```python
from build123d import *

# Parameters (mm, degrees)
F1_DEPTH = 70
F3_DEPTH = 70.001
F5_DEPTH = 5
F7_DEPTH = 5
F6_R     = 2.5
F8_DEPTH = 6


with BuildPart() as f1:
    # F0 (on Front) → F1 (new body)
    with BuildSketch(Plane.XZ):
        Polygon((64.8236190979, 0), (70, 0), (63.1167820899, 25.6885189599), (39.1096145047, 115.2844881338), (34.2799853733, 113.9903929083), (36.2175250532, 106.7593963813), (0, 0), (5.2798833988, 0), (38.5474912469, 98.0638441664), align=None)
    extrude(amount=F1_DEPTH)

    # F2 (on Right) → F3 (cut, through all)
    with BuildSketch(Plane.YZ):
        Polygon((-31.1044628837, 176.4021748616), (0, 0), (48.4349839389, -5.1851687022), (65.811291337, 203.3304870129), align=None)
        Polygon((-111.5468591452, -12.9745472223), (-70, 0), (-38.8955371163, 176.4021748616), (-111.5468591452, 176.4021748616), align=None)
    extrude(amount=F3_DEPTH, mode=Mode.SUBTRACT)

    # F4 (on face) → F5 (cut)
    with BuildSketch(Plane(origin=(0, 0, 0), x_dir=(0, -1, 0), z_dir=(-0.9469906099, 0, 0.3212612407))):
        Polygon((58.1917434691, 10.0000029223), (42.7067823189, 102.7354300022), (27.2932176811, 102.7354300022), (11.8082565309, 10.0000029223), align=None)
    extrude(amount=-F5_DEPTH, mode=Mode.SUBTRACT)

    # F6 (on face) → F7 (cut)
    with BuildSketch(Plane(origin=(65.3108891325, 0, 17.5), x_dir=(0, 1, 0), z_dir=(0.9659258263, 0, 0.2588190451))):
        Polygon((-10.1440055617, -18.1173331572), (-11.8471934071, -8.1173331572), (-14.0249093092, 4.6687838175), (-55.9750906908, 4.6687838175), (-58.1528065929, -8.1173331572), (-59.8559944383, -18.1173331572), align=None)
        Polygon((-26.5845061685, 78.4104846719), (-43.4154938315, 78.4104846719), (-54.3229984458, 14.3687840231), (-15.6770015542, 14.3687840231), align=None)
    extrude(amount=-F7_DEPTH, mode=Mode.SUBTRACT)

    # F6 (on face) → F8 (join)
    with BuildSketch(Plane(origin=(65.3108891325, 0, 17.5), x_dir=(0, 1, 0), z_dir=(0.9659258263, 0, 0.2588190451))):
        with Locations((-60.195499549, 9.6687838175)):
            Circle(F6_R)
        with Locations((-9.804500451, 9.6687838175)):
            Circle(F6_R)
    extrude(amount=F8_DEPTH)


solid = f1.part
```
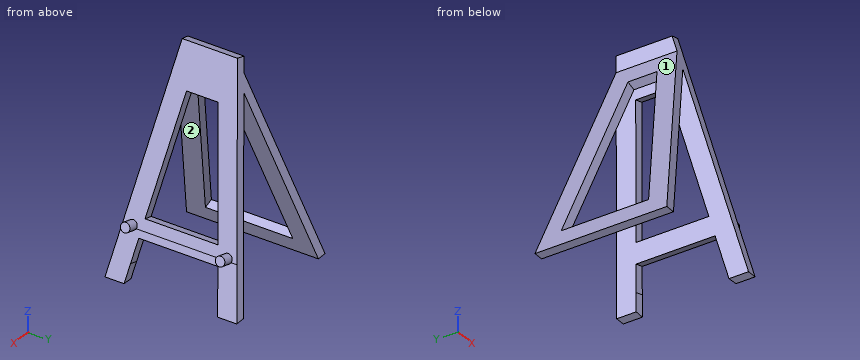
Build history of the part. All positions in model axes, mm. Face numbers are marked on the shaded views. Coordinates: 2 decimals unless noted, no trailing zeros. Order: outer loops, then holes, each group sorted by start corner. A loop starts at its lowest first (then second) coordinate and runs counter-clockwise, first axis right, second up. Notation, with made-up numbers: (67, 40.25) -> (88, 40.25) arc R19 cw to (88, 55.25) -> close; hole circle Ø6 at (1.5, 8.5). An arc over 180 degrees is marked (long way). Answer in a Markdown table with one row per item. Add a question column.
Q1. Band-saw the part on D-D, the plane x = 50.5. List the corners of the cut face in (y, z) (3 decimals), then the cut area to 3 significant figures.
Q2. Wall check: line 1 along X through (y, z) = (-46.5, 93); line 2 along X through (y, z) = (-19, 94); line 3 along Y through (x, z) = (10, 20.5). Give the ranges that are in metal, low to high. Write a range as [from, to].
Q3. Band-saw the part on B-B, the plane x = 27.5. List the corners of the cut face in (y, z).
Q4. Band-saw the part on A-A, the plane y = -34.5. List the corners of the cut face in (x, z).
Q5. Drop flat-ended pins along their axis: pin 1 (5 mm diameter, centred on x = 17, z = 44, fed in from +Y); pin 2 (1.5 mm diameter, centred on y = -27.5, z = 28, fed in from +X); pin 3 (6 mm diameter, centred on x = 15.5, z = 50.5, fed in from -Y). Give the stop position or say it passes through.
Q6. Band-saw the part on C-C, the plane z = 48. List the corners of the cut face in (x, y), then the cut area to 3 significant figures.
Q7. Mould opens along X. For the marked faces 1 and 2 say: +X half, -X half, draft (parallel to the pull), parting line (faces both ways), or undercut.
Answers follow:
| question | item | result |
|---|---|---|
| 1 | outline | (-60.574, 53.456) -> (-50.202, 53.456) -> (-47.024, 72.775) -> (-57.168, 72.775) -> close; (-22.976, 72.775) -> (-19.798, 53.456) -> (-9.426, 53.456) -> (-12.832, 72.775) -> close |
| 1 | area | 396 mm^2 |
| 2 | line 1 | [31.55, 36.83], [39.9, 45.08] |
| 2 | line 2 | [31.89, 37.17], [39.64, 44.81] |
| 2 | line 3 | [-66.39, -56.08], [-13.92, -3.61] |
| 3 | outline | (-58.45, 65.5) -> (-48.03, 65.5) -> (-45.57, 81.06) -> (-55.71, 81.06) -> close; (-24.43, 81.06) -> (-21.97, 65.5) -> (-11.55, 65.5) -> (-14.29, 81.06) -> close |
| 4 | outline | (0, 0) -> (5.28, 0) -> (7.95, 7.86) -> (3.21, 9.47) -> close; (33, 97.29) -> (37.74, 95.68) -> (38.55, 98.06) -> (40.19, 91.94) -> (45.02, 93.24) -> (39.11, 115.28) -> (34.28, 113.99) -> (36.22, 106.76) -> close; (56.76, 30.09) -> (59.27, 20.72) -> (64.1, 22.01) -> (61.59, 31.38) -> close |
| 5 | pin 1 | y = -7.32 |
| 5 | pin 2 | x = 62.7 |
| 5 | pin 3 | y = -61.61 |
| 6 | outline | (16.28, -61.54) -> (21.56, -61.54) -> (21.56, -51.11) -> (16.28, -51.4) -> close; (16.28, -18.6) -> (21.56, -18.89) -> (21.56, -8.46) -> (16.28, -8.46) -> close; (51.96, -61.54) -> (57.14, -61.54) -> (57.14, -51.39) -> (51.96, -51.16) -> close; (51.96, -18.84) -> (57.14, -18.61) -> (57.14, -8.46) -> (51.96, -8.46) -> close |
| 6 | area | 215 mm^2 |
| 7 | face 1 | -X half |
| 7 | face 2 | undercut |
